```python
from build123d import *

# Parameters (mm, degrees)
F1_DEPTH = 18
F2_DEPTH = 2
F3_R     = 3
F4_R     = 1
F5_SIZE  = 1.4


with BuildPart() as f1:
    # F0 (on Top) → F1 (new body)
    with BuildSketch(Plane.XY):
        with BuildLine():
            Line((4.065864, 1.59099), (34.374522, 31.899648))
            ThreePointArc((34.374522, 31.899648), (34.963359, 66.902619), (0, 68.668465))
            ThreePointArc((0, 68.668465), (-34.963359, 66.902619), (-34.374522, 31.899648))
            Line((-34.374522, 31.899648), (-4.065864, 1.59099))
            ThreePointArc((-4.065864, 1.59099), (0, -0.093146), (4.065864, 1.59099))
        make_face()
        with BuildLine():
            ThreePointArc((2.828427, 2.828427), (0, 1.656854), (-2.828427, 2.828427))
            Line((-2.828427, 2.828427), (-33.137085, 33.137085))
            ThreePointArc((-33.137085, 33.137085), (-34.231441, 65.102225), (-2.415992, 68.380169))
            ThreePointArc((-2.415992, 68.380169), (0, 67.568113), (2.415992, 68.380169))
            ThreePointArc((2.415992, 68.380169), (34.231441, 65.102225), (33.137085, 33.137085))
            Line((33.137085, 33.137085), (2.828427, 2.828427))
        make_face(mode=Mode.SUBTRACT)
    extrude(amount=F1_DEPTH)

    # F0 (on Top) → F2 (join)
    with BuildSketch(Plane.XY):
        with BuildLine():
            Line((-36.672619, 29.601551), (-6.363961, -0.707107))
            ThreePointArc((-6.363961, -0.707107), (0, -3.343146), (6.363961, -0.707107))
            Line((6.363961, -0.707107), (36.672619, 29.601551))
            ThreePointArc((36.672619, 29.601551), (38.245177, 68.103217), (0, 72.810414))
            ThreePointArc((0, 72.810414), (-38.245177, 68.103217), (-36.672619, 29.601551))
        make_face()
        with BuildLine():
            ThreePointArc((0, 68.668465), (34.963359, 66.902619), (34.374522, 31.899648))
            Line((34.374522, 31.899648), (4.065864, 1.59099))
            ThreePointArc((4.065864, 1.59099), (0, -0.093146), (-4.065864, 1.59099))
            Line((-4.065864, 1.59099), (-34.374522, 31.899648))
            ThreePointArc((-34.374522, 31.899648), (-34.963359, 66.902619), (0, 68.668465))
        make_face(mode=Mode.SUBTRACT)
    extrude(amount=F2_DEPTH)

    # F3
    f3_edges = [f1.edges().sort_by_distance(p)[0] for p in [
        (0, 68.668465, 10),
    ]]
    fillet(f3_edges, radius=F3_R)

    # F4
    f4_edges = [f1.edges().sort_by_distance(p)[0] for p in [
        (35.715275, 66.061313, 2),
        (38.245177, 68.103217, 2),
        (0, 72.810414, 1),
    ]]
    fillet(f4_edges, radius=F4_R)

    # F5
    f5_edges = [f1.edges().sort_by_distance(p)[0] for p in [
        (35.715275, 66.061313, 18),
    ]]
    chamfer(f5_edges, length=F5_SIZE)


solid = f1.part
```
Input: part model. Units: mm. Frame: model coordinates. A direction names the side the tool comes from. Give positions to 0.01 mm unless a question says otherwise; leave off trailing zeros. Return JSON: item names as keys, results as strings.
Item 1: Access query for faces 4 (the flat face through (18, 18, 9)), 5 (the flat face through (3, 73, 2)), 6 (the flat face through (19.008, 16.533, 9.705)). Directions: +Z, -Z, +X, -X, +Y, -Y. A direction counts if a zero-diameter tool reaches every point of the face in a straight line with its end or side. Return the directions, or none.
Solutions:
{"face 4": "+Z, -Z", "face 5": "+Z", "face 6": "+Z, +X, -Y"}
Item 2: Pull-direction query (X, two-part tool) for faces 1 (the cylindrical face through (-21.093, 14.448, 1.715)), 2 (the cylindrical face through (-0.099, -3.343, 0.493)), 3 (the cylindrical face through (36.05, 65.66, 9.7)); classes: +X half, -X half, draft (parallel to the pull), parting line (faces both ways), or undercut.
Solutions:
{"face 1": "-X half", "face 2": "parting line", "face 3": "undercut"}
Item 3: First-contact query: P1, Ø6, axis at y = 25.5, z = 13, coming from the -X side; P2, Ø5, axis at x = 13.5, z = 15, coming from the -Y side; P3, Ø1.5, axis at y = 42.5, z = 6.5, coming from the +X side. Flat tips, straight axial feed; report the tip coordinate or a pass-through.
Solutions:
{"P1": "x = -30.97", "P2": "y = 8.53", "P3": "x = 40.91"}
Item 4: Ray query, probe 1 along Y at (x, z) = (-19, 6); probe 2 along X at (y, z) = (3, 12); probe 3 along X at (y, z) = (74, 1.5). Return the intervals inside material, ascending.
Solutions:
{"probe 1": "16.53 to 19, 73.01 to 74.77", "probe 2": "-5.47 to -3, 3 to 5.47", "probe 3": "-31.08 to -2.06, 2.06 to 31.08"}
